Study the drawing (mm; zero at the part's minimum x, y, z) and answer. Give positions to 0.01 mm unless a question says otherwise; leave off trailing zeros. Write each loop counter-clockwise with the first axis right and the second up, starting at its lowest first coordinate (ties: lowest second). Pieces come first, ordered by that corner, then holes.
1) Find section C-C (y = 60). Determine the outline of the cut face in (x, z).
2) Straight lines are drawn through the part: probe 1 along Y at (x, z) = (6.5, 1); probe 2 along X at (y, z) = (15, 0.4); probe 3 along Y at (x, z) = (82.5, 1.15). For each, find the intervals that lie inside material, in ascending order.
3) Find section A-A (z = 0.35). Determine the outline of the cut face in (x, y).
4) Given pin 1 Ø1 at (y, z) = (62, 0.5) entering from -X; pin 2 Ø1 at (x, z) = (5.5, 1) entering from -Y; pin 3 Ø0.6 at (x, z) = (3, 1) entering from -Y, each flat-ended and moving along its own axis, determine where each tip first touches the part or whether it passes through.
5) Find section B-B (x = 66). Determine the outline of the cut face in (y, z).
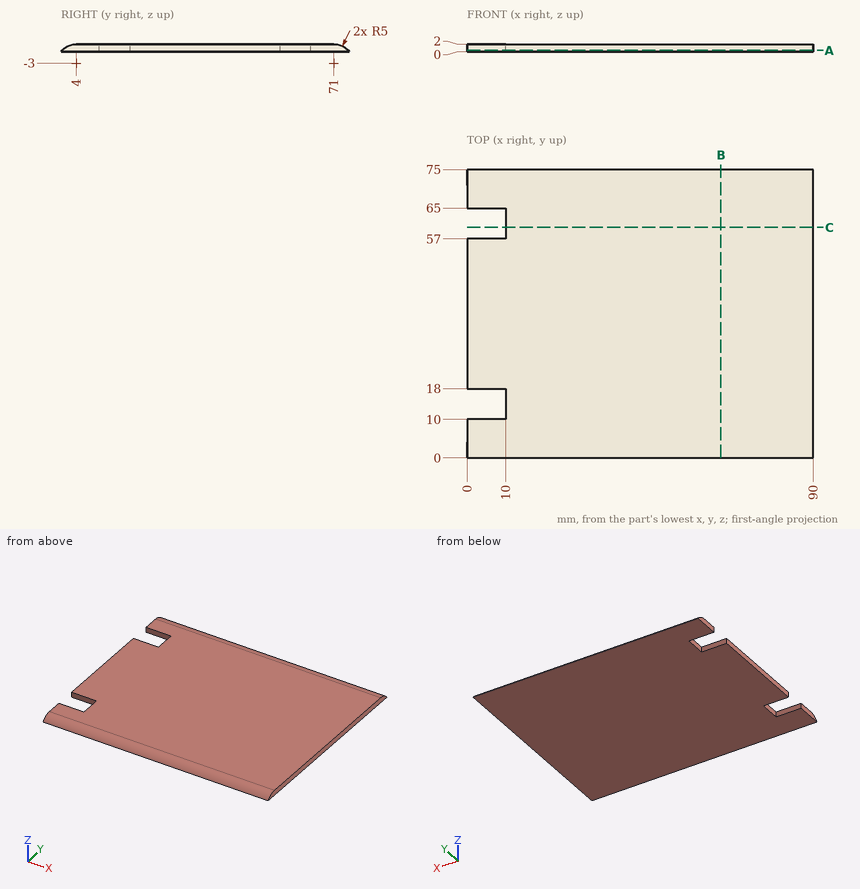
Results:
1. outline: (10, 0) - (90, 0) - (90, 2) - (10, 2) - close
2. probe 1: y = 1 to 10, 18 to 57, 65 to 74
2. probe 2: x = 10 to 90
2. probe 3: y = 1.21 to 73.79
3. outline: (0, 0.29) - (90, 0.29) - (90, 74.71) - (0, 74.71) - (0, 65) - (10, 65) - (10, 57) - (0, 57) - (0, 18) - (10, 18) - (10, 10) - (0, 10) - close
4. pin 1: stops at x = 10
4. pin 2: stops at y = 0.43
4. pin 3: stops at y = 0.64
5. outline: (0, 0) - (75, 0) arc R5 ccw to (71, 2) - (4, 2) arc R5 ccw to start
